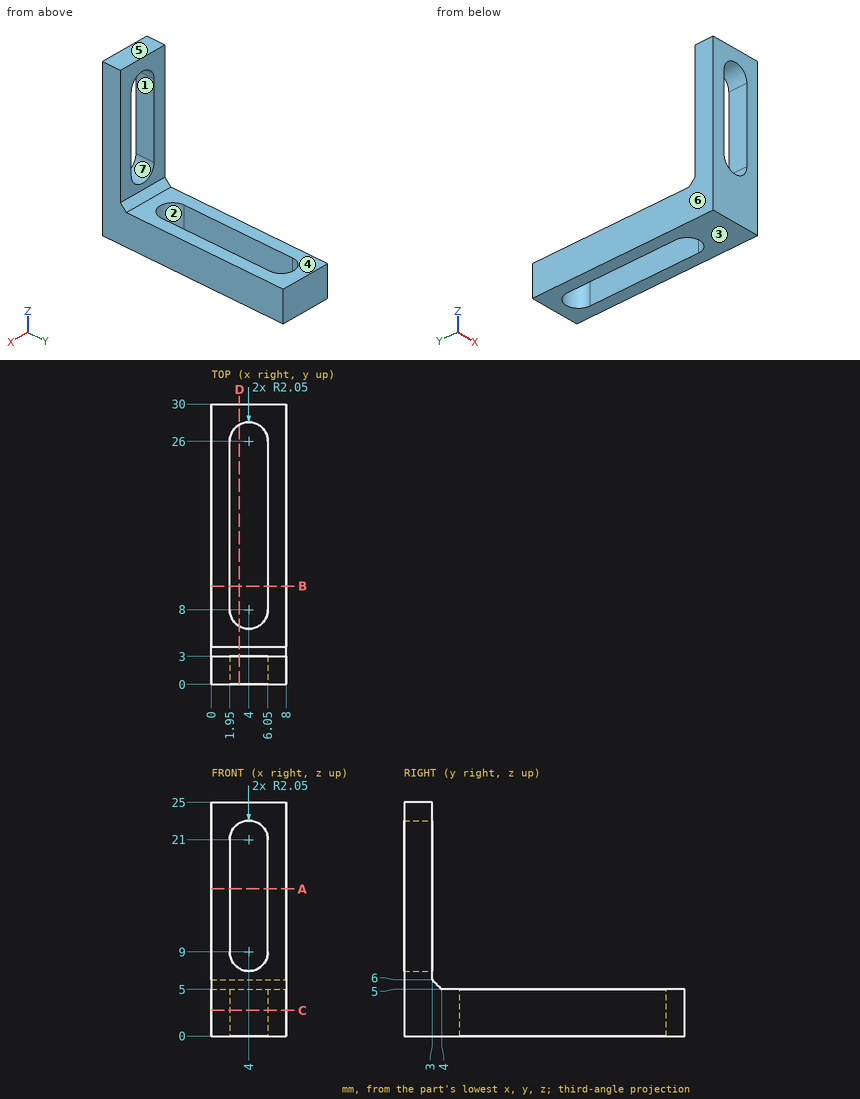
Study the drawing (mm; zero at the part's minimum x, y, z) and answer. A direction names the side the tool comes from. Give positions to 0.01 mm unless a question says otherwise; leave off trailing zeros. Order: outer loops, then holes, each group sorted by start corner. A loop starts at its lowest first (then second) coordinate and runs counter-clockwise, first axis right, second up.
1) Find section A-A on z = 15.75. Write down the section's boundary in (x, y).
Reported:
outline: (0, 0) - (1.95, 0) - (1.95, 3) - (0, 3) - close; (6.05, 0) - (8, 0) - (8, 3) - (6.05, 3) - close
2) Find section B-B on y = 10.5. Write down the section's boundary in (x, z), then the cut area to 3 significant figures.
Reported:
outline: (0, 0) - (1.95, 0) - (1.95, 5) - (0, 5) - close; (6.05, 0) - (8, 0) - (8, 5) - (6.05, 5) - close
area: 19.5 mm2
3) Consider line 1 along Z through (x, y) = (0.5, 26.75); line 2 along Y through (x, z) = (7, 13.25); line 3 along X through (y, z) = (27.5, 3.5). Determine where each line is inside the solid, lowest interval first.
Reported:
line 1: z = 0 to 5
line 2: y = 0 to 3
line 3: x = 0 to 2.6, 5.4 to 8
4) Find section C-C on z = 2.75. Write down the section's boundary in (x, y), then the cut area to 3 significant figures.
Reported:
outline: (0, 0) - (8, 0) - (8, 30) - (0, 30) - close; hole (1.95, 8) arc R2.05 ccw to (6.05, 8) - (6.05, 26) arc R2.05 ccw to (1.95, 26) - close
area: 153 mm2
5) Find section D-D on x = 3. Write down the section's boundary in (y, z), then the cut area to 3 significant figures.
Reported:
outline: (0, 0) - (6.21, 0) - (6.21, 5) - (4, 5) - (3, 6) - (3, 7.21) - (0, 7.21) - close; (0, 22.79) - (3, 22.79) - (3, 25) - (0, 25) - close; (27.79, 0) - (30, 0) - (30, 5) - (27.79, 5) - close
area: 55.9 mm2
6) For the marked faces 1, 2, 3 and 4, determine the directions among +Z, -Z, +X, -X, +Y, -Y from which every point of the face is accessible in a straight line to the end or side of a thin tool.
Reported:
face 1: +Y, -Y
face 2: +Z, -Z
face 3: -Z, +X, -X, +Y, -Y
face 4: +Z, +X, -X, +Y
7) Given P1, Ø2.5, axis at x = 6, y = 13, coming from the +Z side; P2, Ø1.5, axis at x = 3.5, z = 7.5, coming from the +Y side, each flat-ended and moving along its own axis, determine where each tip first touches the part or whether it passes through.
Reported:
P1: stops at z = 5
P2: stops at y = 3
8) Determine the mould class of the marked faces 5, 6 and 7 for opening direction X: pulls with the +X half, pulls with the -X half, needs draft (parallel to the pull), parting line crosses it, or undercut.
Reported:
face 5: needs draft
face 6: pulls with the -X half
face 7: undercut
